Can you work these out from the model? Positions are in its coordinate system, mm. A direction names the side the tool comes from. Give positions to 0.01 mm unless a question says otherwise; leave off trailing zeros. Write each loop counter-clockwise with the first axis right and the second up, starting at its lowest first coordinate (ties: lowest second). Pieces come first, ordered by that corner, then holes.
```python
from build123d import *

# Parameters (mm, degrees)
F1_DEPTH        = 25
F2_DEPTH        = 10
F3_DEPTH        = 20
F4_DEPTH        = 30
F5_R            = 7.49999
F6_SIZE         = 5
F7_R            = 10
F8_DEPTH        = 10
F10_D           = 14.75
F10_CBORE_D     = 22.25
F10_CBORE_DEPTH = 14


# Not quite as in the source:
# - a fillet or chamfer is up to 0.001 mm smaller than in the source, because OpenCascade refuses the exact size


with BuildPart() as f1:
    # F0 (on Front) → F1 (new body)
    with BuildSketch(Plane.XZ):
        with BuildLine():
            Line((96.5, 100), (-96.5, 100))
            ThreePointArc((-96.5, 100), (-103.5710678119, 97.0710678119), (-106.5, 90))
            Line((-106.5, 90), (-106.5, -90))
            ThreePointArc((-106.5, -90), (-103.5710678119, -97.0710678119), (-96.5, -100))
            Line((-96.5, -100), (-63.5, -100))
            Line((-63.5, -100), (-63.5, -43.2740040786))
            ThreePointArc((-63.5, -43.2740040786), (-57.9897187751, -27.6167098657), (-43.8879310345, -18.8615031996))
            ThreePointArc((-43.8879310345, -18.8615031996), (0.846717088, 5.653282912), (25.3615031996, 50.3879310345))
            ThreePointArc((25.3615031996, 50.3879310345), (34.1167098657, 64.4897187751), (49.7740040786, 70))
            Line((49.7740040786, 70), (106.5, 70))
            Line((106.5, 70), (106.5, 90))
            ThreePointArc((106.5, 90), (103.5710678119, 97.0710678119), (96.5, 100))
        make_face()
        with BuildLine():
            ThreePointArc((17.5, 70), (-6.2243507239, 12.7243507239), (-63.5, -11))
            Line((-63.5, -11), (-87.5, -11))
            ThreePointArc((-87.5, -11), (-94.5710678119, -8.0710678119), (-97.5, -1))
            Line((-97.5, -1), (-97.5, 81))
            ThreePointArc((-97.5, 81), (-94.5710678119, 88.0710678119), (-87.5, 91))
            Line((-87.5, 91), (7.5, 91))
            ThreePointArc((7.5, 91), (14.5710678119, 88.0710678119), (17.5, 81))
            Line((17.5, 81), (17.5, 70))
        make_face(mode=Mode.SUBTRACT)
        with BuildLine():
            ThreePointArc((-96.5, -100), (-103.5710678119, -97.0710678119), (-106.5, -90))
            Line((-106.5, -90), (-106.5, -100))
            Line((-106.5, -100), (-96.5, -100))
        make_face()
        with BuildLine():
            Line((106.5, 55), (106.5, 70))
            Line((106.5, 70), (49.7740040786, 70))
            ThreePointArc((49.7740040786, 70), (34.1167098657, 64.4897187751), (25.3615031996, 50.3879310345))
            ThreePointArc((25.3615031996, 50.3879310345), (0.846717088, 5.653282912), (-43.8879310345, -18.8615031996))
            ThreePointArc((-43.8879310345, -18.8615031996), (-57.9897187751, -27.6167098657), (-63.5, -43.2740040786))
            Line((-63.5, -43.2740040786), (-63.5, -100))
            Line((-63.5, -100), (-48.5, -100))
            Line((-48.5, -100), (-48.5, -43.2740040786))
            ThreePointArc((-48.5, -43.2740040786), (-46.29588751, -37.0110863935), (-40.6551724138, -33.509003727))
            ThreePointArc((-40.6551724138, -33.509003727), (11.4533188058, -4.9533188058), (40.009003727, 47.1551724138))
            ThreePointArc((40.009003727, 47.1551724138), (43.5110863935, 52.79588751), (49.7740040786, 55))
            Line((49.7740040786, 55), (106.5, 55))
        make_face()
        with BuildLine():
            Line((106.5, -40), (106.5, 55))
            Line((106.5, 55), (49.7740040786, 55))
            ThreePointArc((49.7740040786, 55), (43.5110863935, 52.79588751), (40.009003727, 47.1551724138))
            ThreePointArc((40.009003727, 47.1551724138), (11.4533188058, -4.9533188058), (-40.6551724138, -33.509003727))
            ThreePointArc((-40.6551724138, -33.509003727), (-46.29588751, -37.0110863935), (-48.5, -43.2740040786))
            Line((-48.5, -43.2740040786), (-48.5, -100))
            Line((-48.5, -100), (46.5, -100))
            Line((46.5, -100), (46.5, -55))
            ThreePointArc((46.5, -55), (50.8933982822, -44.3933982822), (61.5, -40))
            Line((61.5, -40), (106.5, -40))
        make_face()
        with BuildLine():
            Line((56.7871564216, 46), (87.5, 46))
            ThreePointArc((87.5, 46), (94.5710678119, 43.0710678119), (97.5, 36))
            Line((97.5, 36), (97.5, -21))
            ThreePointArc((97.5, -21), (94.5710678119, -28.0710678119), (87.5, -31))
            Line((87.5, -31), (61.5, -31))
            ThreePointArc((61.5, -31), (44.5294372515, -38.0294372515), (37.5, -55))
            Line((37.5, -55), (37.5, -81))
            ThreePointArc((37.5, -81), (34.5710678119, -88.0710678119), (27.5, -91))
            Line((27.5, -91), (-29.5, -91))
            ThreePointArc((-29.5, -91), (-36.5710678119, -88.0710678119), (-39.5, -81))
            Line((-39.5, -81), (-39.5, -50.2871564216))
            ThreePointArc((-39.5, -50.2871564216), (-37.474960815, -44.25391517), (-32.22, -40.6641839079))
            ThreePointArc((-32.22, -40.6641839079), (17.8172798365, -11.3172798365), (47.1641839079, 38.72))
            ThreePointArc((47.1641839079, 38.72), (50.75391517, 43.974960815), (56.7871564216, 46))
        make_face(mode=Mode.SUBTRACT)
        with BuildLine():
            Line((106.5, -90), (106.5, -40))
            Line((106.5, -40), (61.5, -40))
            ThreePointArc((61.5, -40), (50.8933982822, -44.3933982822), (46.5, -55))
            Line((46.5, -55), (46.5, -100))
            Line((46.5, -100), (96.5, -100))
            ThreePointArc((96.5, -100), (97.0006277506, -99.9874607311), (97.5, -99.9498743711))
            ThreePointArc((97.5, -99.9498743711), (103.5710678119, -97.0710678119), (106.4498743711, -91))
            ThreePointArc((106.4498743711, -91), (106.4874607311, -90.5006277506), (106.5, -90))
        make_face()
        with BuildLine():
            Line((106.5, -91), (106.5, -90))
            ThreePointArc((106.5, -90), (106.4874607311, -90.5006277506), (106.4498743711, -91))
            Line((106.4498743711, -91), (106.5, -91))
        make_face()
        with BuildLine():
            Line((106.5, -91), (106.4498743711, -91))
            ThreePointArc((106.4498743711, -91), (103.5710678119, -97.0710678119), (97.5, -99.9498743711))
            Line((97.5, -99.9498743711), (97.5, -100))
            Line((97.5, -100), (106.5, -100))
            Line((106.5, -100), (106.5, -91))
        make_face()
        with BuildLine():
            ThreePointArc((97.5, -99.9498743711), (97.0006277506, -99.9874607311), (96.5, -100))
            Line((96.5, -100), (97.5, -100))
            Line((97.5, -100), (97.5, -99.9498743711))
        make_face()
        with BuildLine():
            Line((-87.5, -11), (-63.5, -11))
            ThreePointArc((-63.5, -11), (-6.2243507239, 12.7243507239), (17.5, 70))
            Line((17.5, 70), (17.5, 81))
            ThreePointArc((17.5, 81), (14.5710678119, 88.0710678119), (7.5, 91))
            Line((7.5, 91), (-87.5, 91))
            ThreePointArc((-87.5, 91), (-94.5710678119, 88.0710678119), (-97.5, 81))
            Line((-97.5, 81), (-97.5, -1))
            ThreePointArc((-97.5, -1), (-94.5710678119, -8.0710678119), (-87.5, -11))
        make_face()
        with BuildLine():
            ThreePointArc((97.5, 36), (94.5710678119, 43.0710678119), (87.5, 46))
            Line((87.5, 46), (56.7871564216, 46))
            ThreePointArc((56.7871564216, 46), (50.75391517, 43.974960815), (47.1641839079, 38.72))
            ThreePointArc((47.1641839079, 38.72), (17.8172798365, -11.3172798365), (-32.22, -40.6641839079))
            ThreePointArc((-32.22, -40.6641839079), (-37.474960815, -44.25391517), (-39.5, -50.2871564216))
            Line((-39.5, -50.2871564216), (-39.5, -81))
            ThreePointArc((-39.5, -81), (-36.5710678119, -88.0710678119), (-29.5, -91))
            Line((-29.5, -91), (27.5, -91))
            ThreePointArc((27.5, -91), (34.5710678119, -88.0710678119), (37.5, -81))
            Line((37.5, -81), (37.5, -55))
            ThreePointArc((37.5, -55), (44.5294372515, -38.0294372515), (61.5, -31))
            Line((61.5, -31), (87.5, -31))
            ThreePointArc((87.5, -31), (94.5710678119, -28.0710678119), (97.5, -21))
            Line((97.5, -21), (97.5, 36))
        make_face()
    extrude(amount=-F1_DEPTH)

    # F0 (on Front) → F2 (join)
    with BuildSketch(Plane.XZ):
        with BuildLine():
            Line((-87.5, -11), (-63.5, -11))
            ThreePointArc((-63.5, -11), (-6.2243507239, 12.7243507239), (17.5, 70))
            Line((17.5, 70), (17.5, 81))
            ThreePointArc((17.5, 81), (14.5710678119, 88.0710678119), (7.5, 91))
            Line((7.5, 91), (-87.5, 91))
            ThreePointArc((-87.5, 91), (-94.5710678119, 88.0710678119), (-97.5, 81))
            Line((-97.5, 81), (-97.5, -1))
            ThreePointArc((-97.5, -1), (-94.5710678119, -8.0710678119), (-87.5, -11))
        make_face()
    extrude(amount=F2_DEPTH)

    # F0 (on Front) → F3 (cut)
    with BuildSketch(Plane.XZ):
        with BuildLine():
            ThreePointArc((97.5, 36), (94.5710678119, 43.0710678119), (87.5, 46))
            Line((87.5, 46), (56.7871564216, 46))
            ThreePointArc((56.7871564216, 46), (50.75391517, 43.974960815), (47.1641839079, 38.72))
            ThreePointArc((47.1641839079, 38.72), (17.8172798365, -11.3172798365), (-32.22, -40.6641839079))
            ThreePointArc((-32.22, -40.6641839079), (-37.474960815, -44.25391517), (-39.5, -50.2871564216))
            Line((-39.5, -50.2871564216), (-39.5, -81))
            ThreePointArc((-39.5, -81), (-36.5710678119, -88.0710678119), (-29.5, -91))
            Line((-29.5, -91), (27.5, -91))
            ThreePointArc((27.5, -91), (34.5710678119, -88.0710678119), (37.5, -81))
            Line((37.5, -81), (37.5, -55))
            ThreePointArc((37.5, -55), (44.5294372515, -38.0294372515), (61.5, -31))
            Line((61.5, -31), (87.5, -31))
            ThreePointArc((87.5, -31), (94.5710678119, -28.0710678119), (97.5, -21))
            Line((97.5, -21), (97.5, 36))
        make_face()
    extrude(amount=-F3_DEPTH, mode=Mode.SUBTRACT)

    # F0 (on Front) → F4 (join)
    with BuildSketch(Plane.XZ):
        with BuildLine():
            Line((106.5, 55), (106.5, 70))
            Line((106.5, 70), (49.7740040786, 70))
            ThreePointArc((49.7740040786, 70), (34.1167098657, 64.4897187751), (25.3615031996, 50.3879310345))
            ThreePointArc((25.3615031996, 50.3879310345), (0.846717088, 5.653282912), (-43.8879310345, -18.8615031996))
            ThreePointArc((-43.8879310345, -18.8615031996), (-57.9897187751, -27.6167098657), (-63.5, -43.2740040786))
            Line((-63.5, -43.2740040786), (-63.5, -100))
            Line((-63.5, -100), (-48.5, -100))
            Line((-48.5, -100), (-48.5, -43.2740040786))
            ThreePointArc((-48.5, -43.2740040786), (-46.29588751, -37.0110863935), (-40.6551724138, -33.509003727))
            ThreePointArc((-40.6551724138, -33.509003727), (11.4533188058, -4.9533188058), (40.009003727, 47.1551724138))
            ThreePointArc((40.009003727, 47.1551724138), (43.5110863935, 52.79588751), (49.7740040786, 55))
            Line((49.7740040786, 55), (106.5, 55))
        make_face()
    extrude(amount=F4_DEPTH)

    # F5 (radius 7.5 in the source; OpenCascade refuses exactly that, so slightly less here)
    f5_edges = [f1.edges().sort_by_distance(p)[0] for p in [
        (-63.5, -30, -71.637002),
        (-48.5, -30, -71.637002),
    ]]
    fillet(f5_edges, radius=F5_R)

    # F6
    f6_edges = [f1.edges().sort_by_distance(p)[0] for p in [
        (-97.5, -10, 40),
    ]]
    chamfer(f6_edges, length=F6_SIZE)

    # F7
    f7_edges = [f1.edges().sort_by_distance(p)[0] for p in [
        (-106.5, 12.5, -100),
        (106.5, 12.5, -100),
    ]]
    fillet(f7_edges, radius=F7_R)

    # F0 (on Front) → F8 (join)
    with BuildSketch(Plane.XZ):
        with BuildLine():
            Line((106.5, -90), (106.5, -40))
            Line((106.5, -40), (61.5, -40))
            ThreePointArc((61.5, -40), (50.8933982822, -44.3933982822), (46.5, -55))
            Line((46.5, -55), (46.5, -100))
            Line((46.5, -100), (96.5, -100))
            ThreePointArc((96.5, -100), (97.0006277506, -99.9874607311), (97.5, -99.9498743711))
            ThreePointArc((97.5, -99.9498743711), (103.5710678119, -97.0710678119), (106.4498743711, -91))
            ThreePointArc((106.4498743711, -91), (106.4874607311, -90.5006277506), (106.5, -90))
        make_face()
    extrude(amount=F8_DEPTH)

    # F10 (through all)
    with Locations(Plane.XZ.offset(10)):
        with Locations((76.5, -70)):
            CounterBoreHole(F10_D / 2, F10_CBORE_D / 2, F10_CBORE_DEPTH)


solid = f1.part
```
1) Please list where these lines run through material, in increasing order: L1, parallel to Z at x = 76.5, y = -3.5 (3 decimals); L2, parallel to Z at x = 76.5, y = 19.75 (3 decimals); L3, parallel to Y at x = 67, z = -59.
Values follow:
L1: z = -100 to -81.125, -58.875 to -40, 55 to 70
L2: z = -100 to -77.375, -62.625 to -31, 46 to 100
L3: y = -10 to 25
2) For faces 1 (the face through (-94.49, -2.46, 88.15)), 2 (the face through (-10.184, -9.757, 15.499)), 3 (the face through (10.9, -11.1, -5.5)), which set-ups out of +Z, -Z, +X, -X, +Y, -Y let a thin tool reach every point of the face, with its end or its side?
Values follow:
face 1: +Z, -X, -Y
face 2: -Y
face 3: -Z, +X, -Y
3) Suppose I cut it at D-D on y = -15. Write out the boundary of the cut face in (x, z).
Values follow:
outline: (-63.5, -100) - (-48.5, -100) - (-48.5, -43.27) arc R10 cw to (-40.66, -33.51) arc R106 ccw to (40.01, 47.16) arc R10 cw to (49.77, 55) - (106.5, 55) - (106.5, 70) - (49.77, 70) arc R25 ccw to (25.36, 50.39) arc R91 cw to (-43.89, -18.86) arc R25 ccw to (-63.5, -43.27) - close
4) For pin 1 Ø2.5 at (y, z) = (-2.5, 48.5) entering from -X; pin 2 Ø11.5 at (x, y) = (78, -13.5) entering from +Z; pin 3 Ø8 at (x, y) = (18, -15) entering from -Z; pin 4 Ø11 at (y, z) = (-3.5, -76) entering from -X, each with a flat end and sliding along its axis, tell me the tip position at first contact or that it passes through.
Values follow:
pin 1: stops at x = -97.5
pin 2: stops at z = 70
pin 3: stops at z = -2.32
pin 4: stops at x = -106.5
5) Suppose I cut it at C-C on z = 72.5. Write out the boundary of the cut face in (x, y).
Values follow:
outline: (-106.5, 0) - (-97.5, 0) - (-97.5, -5) - (-92.5, -10) - (12.5, -10) - (17.5, -5) - (17.5, 0) - (106.5, 0) - (106.5, 25) - (-106.5, 25) - close
